Check sheet for the modelled part. Datum: model origin and axes. Units: mm. A direction names the side the tool comes from. Coordinates: 2 decimals unless noted, no trailing zeros. Order: outer loops, then holes, each group sorted by start corner. A loop starts at its lowest first (then second) coordinate and runs counter-clockwise, first axis right, second up.
1. Cross-section at D-D (z = 0). Enter the section's corners in (x, y), then the cut area to 3 significant figures.
2. Thickness scan on line 1 (Z direction, x = 0, y = 6); line 2 (X direction, y = 118.5, z = -9.5); line 3 (X direction, y = 3.5, z = 0). Record the ranges inside material, lowest first.
3. Cross-section at C-C (z = 9.5). Enter the section's corners in (x, y), then the cut area to 3 significant figures.
4. Cross-section at B-B (y = 107.5). Enter the section's corners in (x, z), then the cut area to 3 significant figures.
5. Cross-section at A-A (x = 0). Enter the section's corners in (y, z).
6. Draft check along Z on faces 1 (the flat face through (-33, 47, -5)), 2 (the flat face through (-40, 72, 0)), 3 (the cylindrical face through (-34.93, 96.653, 1.826)). Enter one of: released by +Z, released by -Z, zero draft, split by the parting line, or undercut.
7. Set-up check for faces 4 (the flat face through (11.5, 10, -0.2)), 5 (the flat face through (-33, 47, 5)), 6 (the flat face through (-2, 0, 11)): record each of +Z, -Z, +X, -X, +Y, -Y from which the full face is reachable in a straight line by a thin tool's end or side.
8. Gauge pin test, flat ends, axial feed: pin 1 Ø1.5 at (y, z) = (13.5, -4) entering from -X; pin 2 Ø5 at (y, z) = (42, 4.5) entering from +X; pin 3 Ø2 at (x, z) = (-32, 5.5) entering from +Y. Record the tip position at first contact, or that the pin passes through.
Autodesk Inventor part; units mm, degrees
ref_plane "YZ Plane" through (0, 0, 0) normal (1, 0, 0) x (0, 1, 0)
ref_plane "XZ Plane" through (0, 0, 0) normal (0, 1, 0) x (-1, 0, 0)
ref_plane "XY Plane" through (0, 0, 0) normal (0, 0, 1) x (1, 0, 0)
sketch "Szkic2" plane through (0, 0, 0) normal (0, 1, 0) x (-1, 0, 0)
  circle A0 centre (0, 0) radius 11
  circle A1 centre (0, 0) radius 16
  dimension "d0" = 22
  dimension "d1" = 5
extrude "Wyciągnięcie proste1" add sketch "Szkic2" along normal blind 10
sketch "Szkic4" plane through (0, 0, 0) normal (0, 0, 1) x (1, 0, 0)
  line L0 (0, 0) -> (-30, 0)
  line L1 (-30, 0) -> (-30, 10)
  line L2 (-30, 10) -> (0, 10)
  line L3 (0, 10) -> (0, 0)
  line L4 (-30, 0) -> (-40, 0)
  line L5 (-40, 0) -> (-40, 107.5)
  line L6 (-40, 107.5) -> (-30, 107.5)
  line L7 (-30, 107.5) -> (-30, 0)
  dimension "d7" = 107.5
  dimension "d8" = 30
  dimension "d9" = 10
  dimension "d10" = 10
extrude "Wyciągnięcie proste2" add sketch "Szkic4" along normal mid plane 10
fillet "Zaokrąglenie1" radius 20 2 edges at (-40, 0, 0) (-30, 10, 0)
sketch "Szkic7" plane through (-30, 107.5, 5) normal (1, 0, 0) x (0, 0, -1)
  line L0 (10, 0) -> (0, 0)
  circle A0 centre (5, 0) radius 11
  circle A1 centre (5, 0) radius 16
  point P0 (5, -107.5)
  dimension "d14" = 22
  dimension "d15" = 32
extrude "Wyciągnięcie proste3" add sketch "Szkic7" against normal blind 10
sketch "Szkic8" plane through (0, 10, 0) normal (0, 1, 0) x (1, 0, 0)
  circle A0 centre (0, 0) radius 11
extrude "Wyciągnięcie proste4" cut sketch "Szkic8" against normal blind 10
sketch "Szkic9" plane through (0, 10, 0) normal (0, -1, 0) x (1, 0, 0)
  circle A0 centre (0, 0) radius 11
extrude "Wyciągnięcie proste5" cut sketch "Szkic9" against normal blind 10
sketch "Szkic11" plane through (-30, 30, 5) normal (1, 0, 0) x (0, 0, -1)
  line L0 (10, 77.5) -> (0, 77.5)
  circle A0 centre (5, 77.5) radius 11
  point P0 (5, -30)
extrude "Wyciągnięcie proste6" cut sketch "Szkic11" against normal blind 10
properties part number "Gora-srodek-ramie"
Data:
1. outline: (-40, 20) arc R20 ccw to (-20, 0) - (-11, 0) - (-11, 10.03) arc R20 cw to (-30, 30) - (-30, 96.5) - (-40, 96.5) - close; (-40, 118.5) - (-30, 118.5) - (-30, 123.5) - (-40, 123.5) - close; (11, 0) - (16, 0) - (16, 10) - (11, 10) - close
1. area: 1,250 mm2
2. line 1: z = -16 to -11, 11 to 16
2. line 2: x = -40 to -30
2. line 3: x = -31.3 to -11, 11 to 16
3. outline: (-40, 94.63) - (-30, 94.63) - (-30, 101.95) - (-40, 101.95) - close; (-40, 113.05) - (-30, 113.05) - (-30, 120.37) - (-40, 120.37) - close; (-12.87, 0) - (-5.55, 0) - (-5.55, 10) - (-10, 10) arc R20 cw to (-12.87, 10.21) - close; (5.55, 0) - (12.87, 0) - (12.87, 10) - (5.55, 10) - close
3. area: 293 mm2
4. outline: (-40, -16) - (-30, -16) - (-30, -11) - (-40, -11) - close; (-40, 11) - (-30, 11) - (-30, 16) - (-40, 16) - close
4. area: 100 mm2
5. outline: (0, -16) - (10, -16) - (10, -11) - (0, -11) - close; (0, 11) - (10, 11) - (10, 16) - (0, 16) - close
6. face 1: released by -Z
6. face 2: zero draft
6. face 3: undercut
7. face 4: +Z, -Z, +X, +Y
7. face 5: +Z, -X, -Y
7. face 6: +Z, -Z, +X, -X, -Y
8. pin 1: stops at x = -39.16
8. pin 2: stops at x = -30
8. pin 3: stops at y = 122.85
